Input: part model. Units: mm. Frame: model coordinates. A direction names the side the tool comes from. Give positions to 0.01 mm unless a question says otherwise; leave off trailing zeros. Order: outer loops, then holes, each group sorted by start corner. A loop starts at its lowest first (then second) coordinate and runs counter-clockwise, first axis right, second up.
```python
from build123d import *

# Parameters (mm, degrees)
SKETCH_2_R          = 1.25
CUT_EXTRUDE_1_DEPTH = 10
CUT_EXTRUDE_START   = -60
SKETCH_2_2_R        = 1.25
CUT_EXTRUDE_2_DEPTH = 6
SKETCH_3_OUTSIDE_W  = 33.036
SKETCH_3_OUTSIDE_H  = 33.036
SKETCH_3_OUTSIDE_R  = 8.75
CUT_EXTRUDE_3_DEPTH = 20
SKETCH_4_R          = 5.25
SKETCH_4_R_2        = 4.25
EXTRUDE_1_DEPTH     = 4


with BuildPart() as part:
    # 草图1 → 旋转1 (revolve)
    with BuildSketch(Plane.XY, mode=Mode.PRIVATE) as revolve_1_sk:
        Polygon((-9, 36), (-5.25, 36), (-5.25, 5), (-9, 5), (-9, 0), (-4.25, 0), (-4.25, 60), (-9, 60), align=None)
    revolve(revolve_1_sk.sketch.rotate(Axis((0, 0, 0), (0, 1, 0)), 270), axis=Axis((0, 0, 0), (0, 1, 0)))

    # 草图2 → 切除-拉伸1 (cut)
    with BuildSketch(Plane(origin=(0, 60, 0), x_dir=(1, 0, 0), z_dir=(0, 1, 0))):
        with Locations(Location((0, 7, 0), (0, 0, 270))):
            Circle(SKETCH_2_R)
        with Locations(Location((0, -7, 0), (0, 0, 270))):
            Circle(SKETCH_2_R)
        with Locations(Location((-7, 0, 0), (0, 0, 270))):
            Circle(SKETCH_2_R)
        with Locations(Location((7, 0, 0), (0, 0, 270))):
            Circle(SKETCH_2_R)
    extrude(amount=-CUT_EXTRUDE_1_DEPTH, mode=Mode.SUBTRACT)

    # 草图2<2> → 切除-拉伸2 (cut)
    with BuildSketch(Plane(origin=(0, 60, 0), x_dir=(1, 0, 0), z_dir=(0, 1, 0)).offset(CUT_EXTRUDE_START)):
        with Locations(Location((0, 7, 0), (0, 0, 270))):
            Circle(SKETCH_2_2_R)
        with Locations(Location((0, -7, 0), (0, 0, 270))):
            Circle(SKETCH_2_2_R)
        with Locations(Location((-7, 0, 0), (0, 0, 270))):
            Circle(SKETCH_2_2_R)
        with Locations(Location((7, 0, 0), (0, 0, 270))):
            Circle(SKETCH_2_2_R)
    extrude(amount=CUT_EXTRUDE_2_DEPTH, mode=Mode.SUBTRACT)

    # 草图3 outside → 切除-拉伸3 (cut)
    with BuildSketch(Plane(origin=(0, 60, 0), x_dir=(1, 0, 0), z_dir=(0, 1, 0))):
        Rectangle(SKETCH_3_OUTSIDE_W, SKETCH_3_OUTSIDE_H)
        with Locations(Location((0, 0, 0), (0, 0, 270))):
            Circle(SKETCH_3_OUTSIDE_R, mode=Mode.SUBTRACT)
    extrude(amount=-CUT_EXTRUDE_3_DEPTH, mode=Mode.SUBTRACT)

    # 草图4 → 凸台-拉伸1 (add)
    with BuildSketch(Plane(origin=(0, 60, 0), x_dir=(1, 0, 0), z_dir=(0, 1, 0))):
        with Locations(Location((0, 0, 0), (0, 0, 90))):
            Circle(SKETCH_4_R)
        with Locations(Location((0, 0, 0), (0, 0, 90))):
            Circle(SKETCH_4_R_2, mode=Mode.SUBTRACT)
    extrude(amount=EXTRUDE_1_DEPTH)


solid = part.part
```
1) Line query: probe 1 along X at (y, z) = (4.05, 0); probe 2 along Y at (x, z) = (-6, -1); probe 3 along Z at (x, y) = (-0.25, 8.5). Output: solid intervals per line, ascending.
2) Cut plane A-A (x = 2.5). Return the cut outline in (y, z).
3) Pull-direction query (X, two-part tool) for faces 1 (the face through (4, 36, -4)), 2 (the face through (-7, 50, 0)), 3 (the face through (-2.703, 2.465, -8.584)); classes: pulls with the +X half, pulls with the -X half, needs draft (parallel to the pull), parting line crosses it, or undercut.
4) Cut plane D-D (z = 7). Return the cut outline in (x, y), then the cut area to 3 significant figures.
5) Cut plane C-C (y = 16). Return the cut outline in (x, z), then the cut area to 3 significant figures.
6) Cut plane B-B (z = 2.75). Return the cut outline in (x, y).
7) First-contact query: P1, Ø6, axis at y = 38, z = -6, coming from the -X side; P2, Ø1.5, axis at x = 5.5, z = 7, coming from the +Y side; P3, Ø2, axis at x = -7, z = 0, coming from the -Y side. Flat tips, straight axial feed; report the tip coordinate or a pass-through.
8) Reachability of faces 4 (the face through (-1.6, 20.3, -5)), 5 (the face through (-8.22, 2.46, -0.27)), 6 (the face through (4, 60, 4)) from +Z, -Z, +X, -X, +Y, -Y: full face, straight path, thin tool, end or side. Return the list, or none.
Geometry says:
1. probe 1: x = -9 to -8.25, -5.75 to -4.25, 4.25 to 5.75, 8.25 to 9
1. probe 2: y = 0 to 5, 36 to 60
1. probe 3: z = -5.24 to -4.24, 4.24 to 5.24
2. outline: (0, -8.65) - (5, -8.65) - (5, -4.62) - (36, -4.62) - (36, -8.65) - (40, -8.65) - (40, -8.39) - (60, -8.39) - (60, -4.62) - (64, -4.62) - (64, -3.44) - (0, -3.44) - close; (0, 3.44) - (64, 3.44) - (64, 4.62) - (60, 4.62) - (60, 8.39) - (40, 8.39) - (40, 8.65) - (36, 8.65) - (36, 4.62) - (5, 4.62) - (5, 8.65) - (0, 8.65) - close
3. face 1: needs draft
3. face 2: undercut
3. face 3: parting line crosses it
4. outline: (-5.66, 0) - (-1.25, 0) - (-1.25, 5) - (-5.66, 5) - close; (-5.66, 36) - (5.66, 36) - (5.66, 40) - (5.25, 40) - (5.25, 60) - (1.25, 60) - (1.25, 50) - (-1.25, 50) - (-1.25, 60) - (-5.25, 60) - (-5.25, 40) - (-5.66, 40) - close; (1.25, 0) - (5.66, 0) - (5.66, 5) - (1.25, 5) - close
4. area: 274 mm2
5. outline: circle Ø10.5 at (0, 0); hole circle Ø8.5 at (0, 0)
5. area: 29.8 mm2
6. outline: (-8.57, 0) - (-3.24, 0) - (-3.24, 64) - (-4.47, 64) - (-4.47, 60) - (-8.31, 60) - (-8.31, 40) - (-8.57, 40) - (-8.57, 36) - (-4.47, 36) - (-4.47, 5) - (-8.57, 5) - close; (3.24, 0) - (8.57, 0) - (8.57, 5) - (4.47, 5) - (4.47, 36) - (8.57, 36) - (8.57, 40) - (8.31, 40) - (8.31, 60) - (4.47, 60) - (4.47, 64) - (3.24, 64) - close
7. P1: stops at x = -8.49
7. P2: stops at y = 60
7. P3: stops at y = 36
8. face 4: none
8. face 5: -Y
8. face 6: +Y
